The figure shows three views and two pictorial views of one solid part (mm, origin at its lowest corner). Answer the questions. A direction names the side the tool comes from. Coordinates: 2 decimals unless noted, no trailing zeros. Order: outer loops, then holes, each group sorted by start corner. A loop starts at its lowest first (then second) coordinate and runs counter-clockwise, first axis right, second up. Notation, with made-up numbers: (50.25, -19.75) -> (61.25, -19.75) arc R32 ccw to (61.25, 8.25) -> close; hole circle Ø5 at (30, 1.25). An arc over 180 degrees is marked (long way). Write item = value, one per line. Start each with the question number.
Q1. Straight lines are drawn through the part: L1, parallel to Z at x = 1.2, y = 4.25; L2, parallel to Z at x = 2.7, y = 1.65; L3, parallel to X at y = 4, z = 11. For each, find the intervals that lie inside material, in ascending order. Write a range as from..to.
Q2. The part is cut by section A-A, the plane z = 5. Determine the outline of the cut face in (x, y).
Q3. For a pull along Y with two mould halves and no side action, classify the marked faces 1, 2 and 3 as +Y half, -Y half, draft (parallel to the pull), parting line (faces both ways), or undercut.
Q4. Flat-ended cylindrical pins translate along their axes: pin 1 (1.5 mm diameter, centred on x = 1, z = 1.5, fed in from +Y); pin 2 (1 mm diameter, centred on x = 4, z = 12, fed in from +Y); pin 3 (3 mm diameter, centred on y = 4, z = 4, fed in from +X). Find the tip coordinate at first contact, or state that the pin passes through.
Q5. Which of the six approach directions +Z, -Z, +X, -X, +Y, -Y give full straight-line access (tool end or side, diameter ignored) to the marked faces 4, 5 and 6?
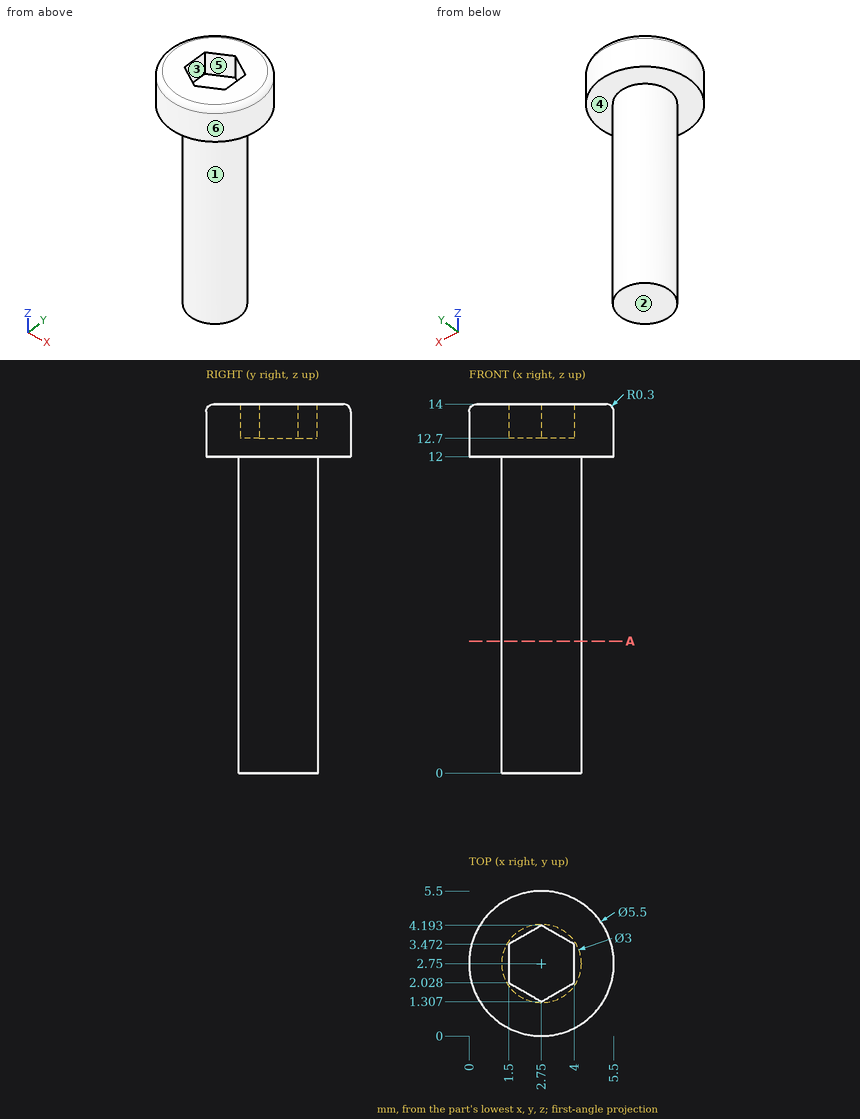
Model answer:
q1.L1 = 12..14
q1.L2 = 0..12.7
q1.L3 = 1.92..3.58
q2.outline = circle Ø3 at (2.75, 2.75)
q3.face_1 = parting line
q3.face_2 = draft
q3.face_3 = undercut
q4.pin_1 = 3.87
q4.pin_2 = 5.4
q4.pin_3 = 4.25
q5.face_4 = -Z
q5.face_5 = +Z
q5.face_6 = +Z, -Z
